Geometry check sheet. Reference: drawing and pictorial views, mm from the part's lowest x, y, z. A direction names the side the tool comes from. Give positions to 0.01 mm unless a question says otherwise; leave off trailing zeros. Order: outer loops, then holes, each group sorted by start corner. A loop starts at its lowest first (then second) coordinate and runs counter-clockwise, first axis right, second up. Notation, with made-up numbers: (14, 77.25) - (68, 77.25) arc R34 cw to (68, 109.25) - close; hole circle Ø9 at (21.5, 14.5). An arc over 180 degrees is marked (long way). Answer in a Markdown table with one row per item.
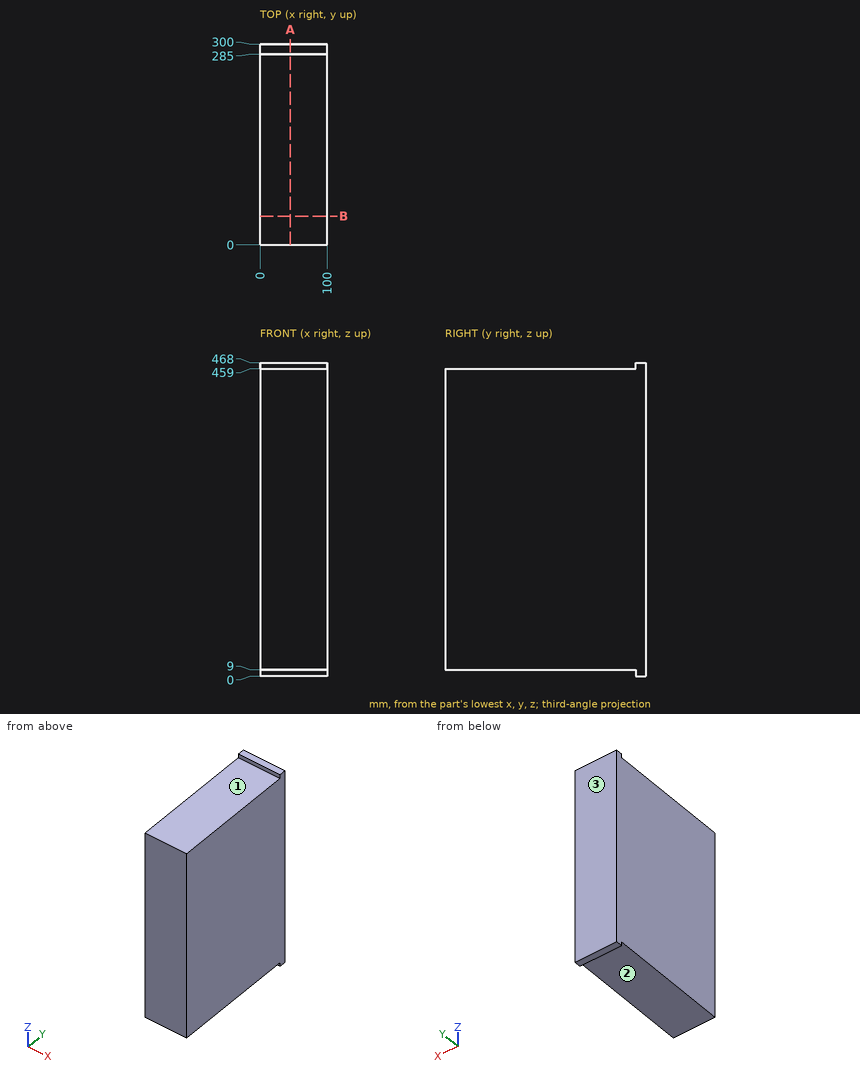
(1) Thickness scan on L1, parallel to Z at x = 65.5, y = 280. Record the ranges inside material, lowest first.
Geometry says:
| item | result |
|---|---|
| L1 | 9 to 459 |
(2) Cross-section at A-A, the plane x = 45. Record the cut outline in (y, z), then the cut area to 3 significant figures.
Geometry says:
| item | result |
|---|---|
| outline | (0, 9) - (285, 9) - (285, 0) - (300, 0) - (300, 468) - (285, 468) - (285, 459) - (0, 459) - close |
| area | 135,000 mm² |
(3) Access from +Z, -Z, +X, -X, +Y, -Y to the whole of each face (thin tool, end or side, straight path). Record for the marked faces 1, 2 and 3.
Geometry says:
| item | result |
|---|---|
| face 1 | +Z, +X, -X, -Y |
| face 2 | -Z, +X, -X, -Y |
| face 3 | +Z, -Z, +X, -X, +Y |
(4) Gauge pin test, flat ends, axial feed: P1, Ø3, axis at x = 42, y = 176, coming from the -Z side; P2, Ø10, axis at x = 78, y = 201, coming from the +Z side; P3, Ø2.5, axis at x = 65.5, z = 465, coming from the -Y side. Record the tip position at first contact, or that the pin passes through.
Geometry says:
| item | result |
|---|---|
| P1 | z = 9 |
| P2 | z = 459 |
| P3 | y = 285 |
(5) Cross-section at B-B, the plane y = 43. Record the cut outline in (x, z), then the cut area to 3 significant figures.
Geometry says:
| item | result |
|---|---|
| outline | (0, 9) - (100, 9) - (100, 459) - (0, 459) - close |
| area | 45,000 mm² |
